Check sheet for the modelled part. Datum: model origin and axes. Units: mm. Face numbers are marked on the shaded views. A direction names the side the tool comes from. Round coordinates to 2 decimals unless told otherwise and drop trailing zeros. Write each loop counter-clockwise with the first axis right and the second up, starting at its lowest first coordinate (ties: lowest second). Pieces come first, ordered by that corner, then holes. Notation, with made-up numbers: (85, -0.5) -> (103, -0.5) arc R29 cw to (103, 36.5) -> close; hole circle Ø1 at (17, 74.25). An arc over 180 degrees is marked (long way). Answer as a JSON object with one key per item and string values. Group by question number.
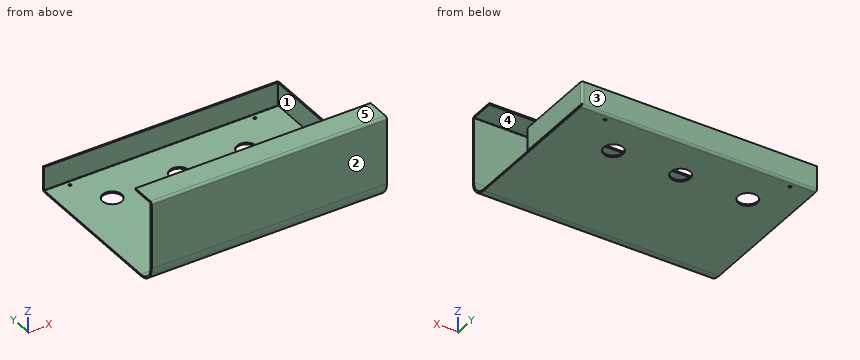
```python
from build123d import *

# Parameters (mm, degrees)
SKETCH_2_W                       = 280
SKETCH_2_H                       = 200
SM_BASE_FLANGE_1_DEPTH           = 2
SM_EDGE_FLANGE_1_STRIP_W         = 44
SM_EDGE_FLANGE_1_STRIP_H         = 2
SM_EDGE_FLANGE_1_STRIP_CUT_DEPTH = 280
SM_EDGE_FLANGE_1_DEPTH           = 280
SM_EDGE_FLANGE_2_STRIP_W         = 9.4732
SM_EDGE_FLANGE_2_STRIP_H         = 2
SM_EDGE_FLANGE_2_STRIP_CUT_DEPTH = 280
SM_EDGE_FLANGE_2_DEPTH           = 280
SM_EDGE_FLANGE_3_STRIP_W         = 9.4732
SM_EDGE_FLANGE_3_STRIP_H         = 2
SM_EDGE_FLANGE_3_STRIP_CUT_DEPTH = 280
SM_EDGE_FLANGE_3_DEPTH           = 280
SKETCH_36_R                      = 11.5
CUT_EXTRUDE_3_DEPTH              = 10
SM_EDGE_FLANGE_4_STRIP_W         = 9.4732
SM_EDGE_FLANGE_4_STRIP_H         = 2
SM_EDGE_FLANGE_4_STRIP_CUT_DEPTH = 27.2634
SM_EDGE_FLANGE_4_DEPTH           = 27.2634
HOLE_WIZARD_M4_1_D               = 3.3


# Sheet-metal steps are written as plain solids
with BuildPart() as part:
    # Sketch 2 → 基体-法兰1 (new body)
    with BuildSketch(Plane.XY):
        Rectangle(SKETCH_2_W, SKETCH_2_H)
    extrude(amount=-SM_BASE_FLANGE_1_DEPTH)

    # 边线-法兰1 strip (across the edge) → 边线-法兰1 strip cut (cut)
    with BuildSketch(Plane(origin=(-140, -100, 0), x_dir=(0, 1, 0), z_dir=(1, 0, 0))):
        with Locations((-2, -1)):
            Rectangle(SM_EDGE_FLANGE_1_STRIP_W, SM_EDGE_FLANGE_1_STRIP_H)
    extrude(amount=SM_EDGE_FLANGE_1_STRIP_CUT_DEPTH, mode=Mode.SUBTRACT)

    # 边线-法兰1 section (across the edge) → 边线-法兰1 (add)
    with BuildSketch(Plane(origin=(-140, -100, 0), x_dir=(0, 1, 0), z_dir=(1, 0, 0))):
        with BuildLine():
            Line((0, 18), (0, 98))
            Line((0, 98), (2, 98))
            Line((2, 98), (2, 18))
            ThreePointArc((2, 18), (7.272077939, 5.272077939), (20, 0))
            Line((20, 0), (20, -2))
            ThreePointArc((20, -2), (5.857864376, 3.857864376), (0, 18))
        make_face()
    extrude(amount=SM_EDGE_FLANGE_1_DEPTH)

    # 边线-法兰2 strip (across the edge) → 边线-法兰2 strip cut (cut)
    with BuildSketch(Plane(origin=(140, 100, 0), x_dir=(0, -1, 0), z_dir=(-1, 0, 0))):
        with Locations((-2, -1)):
            Rectangle(SM_EDGE_FLANGE_2_STRIP_W, SM_EDGE_FLANGE_2_STRIP_H)
    extrude(amount=SM_EDGE_FLANGE_2_STRIP_CUT_DEPTH, mode=Mode.SUBTRACT)

    # 边线-法兰2 section (across the edge) → 边线-法兰2 (add)
    with BuildSketch(Plane(origin=(140, 100, 0), x_dir=(0, -1, 0), z_dir=(-1, 0, 0))):
        with BuildLine():
            Line((0, 0.7366), (0, 28))
            Line((0, 28), (2, 28))
            Line((2, 28), (2, 0.7366))
            ThreePointArc((2, 0.7366), (2.215745145, 0.215745145), (2.7366, 0))
            Line((2.7366, 0), (2.7366, -2))
            ThreePointArc((2.7366, -2), (0.801531583, -1.198468417), (0, 0.7366))
        make_face()
    extrude(amount=SM_EDGE_FLANGE_2_DEPTH)

    # 边线-法兰3 strip (across the edge) → 边线-法兰3 strip cut (cut)
    with BuildSketch(Plane(origin=(-140, -98, 98), x_dir=(0, 0, -1), z_dir=(1, 0, 0))):
        with Locations((-2, -1)):
            Rectangle(SM_EDGE_FLANGE_3_STRIP_W, SM_EDGE_FLANGE_3_STRIP_H)
    extrude(amount=SM_EDGE_FLANGE_3_STRIP_CUT_DEPTH, mode=Mode.SUBTRACT)

    # 边线-法兰3 section (across the edge) → 边线-法兰3 (add)
    with BuildSketch(Plane(origin=(-140, -98, 98), x_dir=(0, 0, -1), z_dir=(1, 0, 0))):
        with BuildLine():
            Line((0, 0.7366), (0, 28))
            Line((0, 28), (2, 28))
            Line((2, 28), (2, 0.7366))
            ThreePointArc((2, 0.7366), (2.215745145, 0.215745145), (2.7366, 0))
            Line((2.7366, 0), (2.7366, -2))
            ThreePointArc((2.7366, -2), (0.801531583, -1.198468417), (0, 0.7366))
        make_face()
    extrude(amount=SM_EDGE_FLANGE_3_DEPTH)

    # 草图36 → 切除-拉伸3 (cut)
    with BuildSketch(Plane(origin=(0, 0, -2), x_dir=(-1, 0, 0), z_dir=(0, 0, -1))):
        with Locations((-70, 50)):
            Circle(SKETCH_36_R)
        with Locations((10, 50)):
            Circle(SKETCH_36_R)
        with Locations((90, 50)):
            Circle(SKETCH_36_R)
    extrude(amount=-CUT_EXTRUDE_3_DEPTH, mode=Mode.SUBTRACT)

    # 边线-法兰4 strip (across the edge) → 边线-法兰4 strip cut (cut)
    with BuildSketch(Plane(origin=(140, 98, 0.7366), x_dir=(-1, 0, 0), z_dir=(0, 0, 1))):
        with Locations((-2, -1)):
            Rectangle(SM_EDGE_FLANGE_4_STRIP_W, SM_EDGE_FLANGE_4_STRIP_H)
    extrude(amount=SM_EDGE_FLANGE_4_STRIP_CUT_DEPTH, mode=Mode.SUBTRACT)

    # 边线-法兰4 section (across the edge) → 边线-法兰4 (add)
    with BuildSketch(Plane(origin=(140, 98, 0.7366), x_dir=(-1, 0, 0), z_dir=(0, 0, 1))):
        with BuildLine():
            Line((0, 0.7366), (0, 98))
            Line((0, 98), (2, 98))
            Line((2, 98), (2, 0.7366))
            ThreePointArc((2, 0.7366), (2.215745145, 0.215745145), (2.7366, 0))
            Line((2.7366, 0), (2.7366, -2))
            ThreePointArc((2.7366, -2), (0.801531583, -1.198468417), (0, 0.7366))
        make_face()
    extrude(amount=SM_EDGE_FLANGE_4_DEPTH)

    # M4 螺纹孔1 (through all)
    with Locations(Plane(origin=(0, 0, -2), x_dir=(-1, 0, 0), z_dir=(0, 0, -1))):
        with Locations((-107, 92), (113, 92)):
            Hole(HOLE_WIZARD_M4_1_D / 2)


solid = part.part
```
(1) Scan lines: line 1 along X through (y, z) = (92, -1); line 2 along Z through (x, y) = (-40.5, -75.5); line 3 along X through (y, z) = (91.5, 8.5). Record each from-to range of solid material in increasing order.
(2) Go/stop test with flat-tipped pins: pin 1 Ø1 at (x, z) = (139, 15) entering from -Y; pin 2 Ø8 at (x, y) = (-50, 50.5) entering from +Z; pin 3 Ø2 at (x, y) = (107, 92) entering from +Z; pin 4 Ø1 at (x, y) = (138.5, 99) entering from +Z. Record where each tip stops, or that it passes through.
(3) Section check A-A on x = -90. Record the cut outline in (y, z).
(4) Section check D-D on y = 50. Record the cut outline in (x, z).
(5) Access from +Z, -Z, +X, -X, +Y, -Y to the whole of each face (thin tool, end or side, straight path). Record for the marked faces 1 and 2.
(6) Section check B-B on y = 80. Record the cut outline in (x, z), then the cut area to 3 significant figures.
(7) Section check C-C on z = 25. Record the cut outline in (x, y), then the cut area to 3 significant figures.
(8) Release check for a two-part mould opening along Z. For the marked faces 3, 4 and 5 record: pulls with the +Z half, pulls with the -Z half, needs draft (parallel to the pull), parting line crosses it, or undercut.
Data:
{
 "1": {"line 1": "x = -140 to -114.65, -111.35 to 105.35, 108.65 to 140", "line 2": "z = -2 to 0, 96 to 98", "line 3": "x = 138 to 140"},
 "2": {"pin 1": "stops at y = -99.84", "pin 2": "stops at z = 0", "pin 3": "passes through", "pin 4": "stops at z = 28"},
 "3": {"outline": "(-100, 18) arc R20 ccw to (-80, -2) -> (38.5, -2) -> (38.5, 0) -> (-80, 0) arc R18 cw to (-98, 18) -> (-98, 95.26) arc R0.74 cw to (-97.26, 96) -> (-70, 96) -> (-70, 98) -> (-97.26, 98) arc R2.74 ccw to (-100, 95.26) -> close; (61.5, -2) -> (97.26, -2) arc R2.74 ccw to (100, 0.74) -> (100, 28) -> (98, 28) -> (98, 0.74) arc R0.74 cw to (97.26, 0) -> (61.5, 0) -> close"},
 "4": {"outline": "(-140, -2) -> (-101.5, -2) -> (-101.5, 0) -> (-140, 0) -> close; (-78.5, -2) -> (-21.5, -2) -> (-21.5, 0) -> (-78.5, 0) -> close; (1.5, -2) -> (58.5, -2) -> (58.5, 0) -> (1.5, 0) -> close; (81.5, -2) -> (140, -2) -> (140, 0) -> (81.5, 0) -> close; (138, 0.74) -> (140, 0.74) -> (140, 28) -> (138, 28) -> close"},
 "5": {"face 1": "+Z, -X", "face 2": "+Z, -Z, +X, -X, -Y"},
 "6": {"outline": "(-140, -2) -> (140, -2) -> (140, 0) -> (-140, 0) -> close; (138, 0.74) -> (140, 0.74) -> (140, 28) -> (138, 28) -> close", "area": "615 mm²"},
 "7": {"outline": "(-140, -100) -> (140, -100) -> (140, -98) -> (-140, -98) -> close; (-140, 98) -> (137.26, 98) arc R0.74 cw to (138, 97.26) -> (138, 0) -> (140, 0) -> (140, 97.26) arc R2.74 ccw to (137.26, 100) -> (-140, 100) -> close", "area": "1,310 mm²"},
 "8": {"face 3": "needs draft", "face 4": "undercut", "face 5": "pulls with the +Z half"}
}
